Source: CAD feature listing. Evaluate the final solid. Frame: model axes, mm. A direction names the side the tool comes from. Give positions to 0.01 mm unless a question says otherwise; leave off trailing zeros. Order: outer loops, then holes, each group sorted by start corner. A loop starts at its lowest first (then second) coordinate and runs counter-clockwise, first axis right, second up. Notation, with made-up numbers: (-29.75, 39.5) -> (3.25, 39.5) arc R18 ccw to (3.25, 73.5) -> close; hole circle Ø11 at (59, -30). An arc over 180 degrees is marked (long way). Answer in a Markdown table with one row per item.
```python
from build123d import *

# Parameters (mm, degrees)
ESQUISSE3_W        = 10
ESQUISSE3_H        = 15
ESQUISSE3_H_2      = 10
ESQUISSE3_H_3      = 5
BOSS_EXTRU_1_DEPTH = 3
ESQUISSE4_W        = 10
ESQUISSE4_H        = 5
ESQUISSE4_H_2      = 3.75
BOSS_EXTRU_2_DEPTH = 17
ESQUISSE5_W        = 20
ESQUISSE5_H        = 18.75
BOSS_EXTRU_4_DEPTH = 4


with BuildPart() as part:
    # Esquisse3 → Boss.-Extru.1 (new body)
    with BuildSketch(Plane(origin=(0, 0, 0), x_dir=(1, 0, 0), z_dir=(0, 1, 0))):
        with Locations((-15.05164944, -6.870348765)):
            Rectangle(ESQUISSE3_W, ESQUISSE3_H)
        with Locations((14.94835056, -6.870348765)):
            Rectangle(ESQUISSE3_W, ESQUISSE3_H)
        with BuildLine():
            Line((-10.05164944, 5.629651235), (-10.05164944, 15.629651235))
            Line((-10.05164944, 15.629651235), (-20.05164944, 15.629651235))
            Line((-20.05164944, 15.629651235), (-20.05164944, 5.629651235))
            Line((-20.05164944, 5.629651235), (-17.25164944, 5.629651235))
            ThreePointArc((-17.25164944, 5.629651235), (-15.05164944, 7.829651235), (-12.85164944, 5.629651235))
            Line((-12.85164944, 5.629651235), (-10.05164944, 5.629651235))
        make_face()
        with BuildLine():
            Line((-10.05164944, 0.629651235), (-10.05164944, 5.629651235))
            Line((-10.05164944, 5.629651235), (-12.85164944, 5.629651235))
            ThreePointArc((-12.85164944, 5.629651235), (-15.05164944, 3.429651235), (-17.25164944, 5.629651235))
            Line((-17.25164944, 5.629651235), (-20.05164944, 5.629651235))
            Line((-20.05164944, 5.629651235), (-20.05164944, 0.629651235))
            Line((-20.05164944, 0.629651235), (-10.05164944, 0.629651235))
        make_face()
        with Locations((-5.05164944, 10.629651235)):
            Rectangle(ESQUISSE3_W, ESQUISSE3_H_2)
        with Locations((4.94835056, 10.629651235)):
            Rectangle(ESQUISSE3_W, ESQUISSE3_H_2)
        with BuildLine():
            Line((19.94835056, 15.629651235), (9.94835056, 15.629651235))
            Line((9.94835056, 15.629651235), (9.94835056, 5.629651235))
            Line((9.94835056, 5.629651235), (12.74835056, 5.629651235))
            ThreePointArc((12.74835056, 5.629651235), (14.94835056, 7.829651235), (17.14835056, 5.629651235))
            Line((17.14835056, 5.629651235), (19.94835056, 5.629651235))
            Line((19.94835056, 5.629651235), (19.94835056, 15.629651235))
        make_face()
        with BuildLine():
            Line((12.74835056, 5.629651235), (9.94835056, 5.629651235))
            Line((9.94835056, 5.629651235), (9.94835056, 0.629651235))
            Line((9.94835056, 0.629651235), (19.94835056, 0.629651235))
            Line((19.94835056, 0.629651235), (19.94835056, 5.629651235))
            Line((19.94835056, 5.629651235), (17.14835056, 5.629651235))
            ThreePointArc((17.14835056, 5.629651235), (14.94835056, 3.429651235), (12.74835056, 5.629651235))
        make_face()
        with Locations((4.94835056, -6.870348765)):
            Rectangle(ESQUISSE3_W, ESQUISSE3_H)
        with Locations((-5.05164944, -6.870348765)):
            Rectangle(ESQUISSE3_W, ESQUISSE3_H)
        with Locations((4.94835056, 3.129651235)):
            Rectangle(ESQUISSE3_W, ESQUISSE3_H_3)
        with Locations((-5.05164944, 3.129651235)):
            Rectangle(ESQUISSE3_W, ESQUISSE3_H_3)
    extrude(amount=BOSS_EXTRU_1_DEPTH)

    # Esquisse4 → Boss.-Extru.2 (add)
    with BuildSketch(Plane(origin=(0, 3, 0), x_dir=(1, 0, 0), z_dir=(0, 1, 0))):
        with Locations((-5.05164944, 3.129651235)):
            Rectangle(ESQUISSE4_W, ESQUISSE4_H)
        with Locations((-5.05164944, -1.245348765)):
            Rectangle(ESQUISSE4_W, ESQUISSE4_H_2)
        with Locations((4.94835056, -1.245348765)):
            Rectangle(ESQUISSE4_W, ESQUISSE4_H_2)
        with Locations((4.94835056, 3.129651235)):
            Rectangle(ESQUISSE4_W, ESQUISSE4_H)
        Polygon((-0.05164944, 15.629651235), (-0.05164944, 5.629651235), (9.94835056, 5.629651235), (9.94835056, 8.129651235), align=None)
        Polygon((-10.05164944, 8.129651235), (-10.05164944, 5.629651235), (-0.05164944, 5.629651235), (-0.05164944, 15.629651235), align=None)
        Polygon((-10.05164944, 15.629651235), (-10.05164944, 8.129651235), (-0.05164944, 15.629651235), align=None)
        Polygon((9.94835056, 15.629651235), (-0.05164944, 15.629651235), (9.94835056, 8.129651235), align=None)
    extrude(amount=BOSS_EXTRU_2_DEPTH)

    # Esquisse5 → Boss.-Extru.4 (add)
    with BuildSketch(Plane(origin=(0, 20, 0), x_dir=(1, 0, 0), z_dir=(0, 1, 0))):
        with Locations((-0.05164944, 6.254651235)):
            Rectangle(ESQUISSE5_W, ESQUISSE5_H)
    extrude(amount=BOSS_EXTRU_4_DEPTH)


solid = part.part
```
(1) Section query D-D (y = 21.75). Return the cut outline in (x, z), plus the area to 3 significant figures.
A:
| item | result |
|---|---|
| outline | (-10.05, -15.63) -> (9.95, -15.63) -> (9.95, 3.12) -> (-10.05, 3.12) -> close |
| area | 375 mm^2 |
(2) Ray query, probe 1 along Y at (x, z) = (-17, 2.25); probe 2 along Z at (x, y) = (-10, 5.75); probe 3 along X at (y, z) = (22.5, 1.25). Return the intervals inside material, ascending.
A:
| item | result |
|---|---|
| probe 1 | y = 0 to 3 |
| probe 2 | z = -15.63 to 3.12 |
| probe 3 | x = -10.05 to 9.95 |
(3) First-contact query: pin 1 Ø5.5 at (y, z) = (12, -10) entering from -X; pin 2 Ø4 at (y, z) = (8, 6.5) entering from -X; pin 3 Ø5 at (x, y) = (-10, 12.5) entering from +Z; pin 4 Ø10 at (x, y) = (12.5, 13.5) entering from -Z. Flat tips, straight axial feed; report the tip coordinate or a pass-through.
A:
| item | result |
|---|---|
| pin 1 | stops at x = -10.05 |
| pin 2 | passes through |
| pin 3 | stops at z = 3.12 |
| pin 4 | stops at z = -15.63 |
(4) Section query A-A (x = 14.5). Return the cut outline in (y, z), plus the area to 3 significant figures.
A:
| item | result |
|---|---|
| outline | (0, -15.63) -> (3, -15.63) -> (3, -7.78) -> (0, -7.78) -> close; (0, -3.48) -> (3, -3.48) -> (3, 14.37) -> (0, 14.37) -> close |
| area | 77.1 mm^2 |
(5) Section query B-B (z = -9.5). Return the cut outline in (x, y).
A:
| item | result |
|---|---|
| outline | (-20.05, 0) -> (19.95, 0) -> (19.95, 3) -> (9.95, 3) -> (9.95, 24) -> (-10.05, 24) -> (-10.05, 3) -> (-20.05, 3) -> close |
(6) Section query C-C (x = 4.5). Return the cut outline in (y, z).
A:
| item | result |
|---|---|
| outline | (0, -15.63) -> (24, -15.63) -> (24, 3.12) -> (3, 3.12) -> (3, 14.37) -> (0, 14.37) -> close |
(7) Access query for faces 1 (the flat face through (-10.052, 13, -6)), 2 (the flat face through (0, 13, 3.12)), 3 (the flat face through (9.948, 13, -6)), 4 (the flat face through (0, 12, -15.63)). Directions: +Z, -Z, +X, -X, +Y, -Y. A direction counts if a zero-diameter tool reaches every point of the face in a straight line with its end or side. Return the directions, or none.
A:
| item | result |
|---|---|
| face 1 | +Z, -Z, -X, +Y |
| face 2 | +Z, +X, -X, +Y |
| face 3 | +Z, -Z, +X, +Y |
| face 4 | -Z, +X, -X, +Y, -Y |
(8) Pull-direction query (Z, two-part tool) for faces 5 (the flat face through (0, 1, 14.37)), 6 (the flat face through (0, 3, 6)), 7 (the cylindrical face through (-13.3, 1.5, -4.3)); classes: +Z half, -Z half, draft (parallel to the pull), parting line (faces both ways), or undercut.
A:
| item | result |
|---|---|
| face 5 | +Z half |
| face 6 | draft |
| face 7 | undercut |
